The listing builds one solid part. Answer for the finished solid, in the listing's coordinates (mm). Round coordinates to 2 decimals unless told otherwise and drop trailing zeros. Write each loop counter-clockwise with the first axis right and the second up, starting at its lowest first coordinate (ties: lowest second). Pieces come first, ordered by that corner, then holes.
(1) A cutting plane is placed at B-B, the plane y = -50. Give the vertices of the cut face in (x, z), and give its area (3 significant figures).
(2) A cutting plane is placed at C-C, the plane x = 10. Give the vertices of the cut face in (y, z).
(3) This flat-tipped pin is pushed along its axis until it touches: pin 1 Ø3.5 at (x, y) = (10, -70) entering from +Z. Where does it stop, or does it pass through?
(4) A cutting plane is placed at A-A, the plane z = -1.5. Give the vertices of the cut face in (x, y).
(5) A cutting plane is placed at D-D, the plane y = -10. Give the vertices of the cut face in (x, z), and give its area (3 significant figures).
(6) Find the intervals of material crossed by probe 1 along X at (y, z) = (-70, -0.65); probe 2 along Y at (x, z) = (10, -0.7); probe 3 along Y at (x, z) = (8, -1.9), in increasing order.
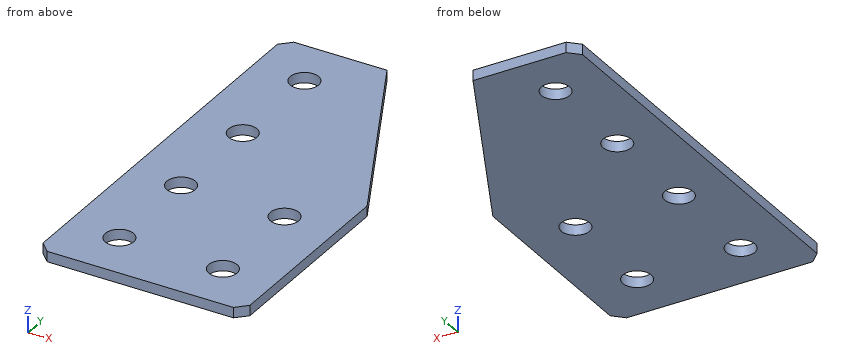
from build123d import *

# Parameters (mm, degrees)
EXTRUDE_1_DEPTH   = 2
HOLE_WIZARD_M51_D = 5.5
CHAMFER_1_SIZE    = 2


with BuildPart() as part:
    # Эскиз1 → Бобышка-Вытянуть1 (new body)
    with BuildSketch(Plane(origin=(0, 0, 0), x_dir=(1, 0, 0), z_dir=(0, 0, -1))):
        Polygon((0, 0), (0, 80), (40, 80), (40, 40), (20, 0), align=None)
    extrude(amount=EXTRUDE_1_DEPTH)

    # Отверстие с зазором M51 (through all)
    with Locations(Plane(origin=(0, 0, -2), x_dir=(1, 0, 0), z_dir=(0, 0, -1))):
        with Locations((10, 70), (10, 50), (10, 30), (10, 10), (30, 70), (30, 50)):
            Hole(HOLE_WIZARD_M51_D / 2)

    # Фаска1
    chamfer_1_edges = [part.edges().sort_by_distance(p)[0] for p in [
        (0, 0, -1),
        (0, -80, -1),
        (40, -80, -1),
    ]]
    chamfer(chamfer_1_edges, length=CHAMFER_1_SIZE)


solid = part.part
Solutions:
1. outline: (0, -2) - (7.25, -2) - (7.25, 0) - (0, 0) - close; (12.75, -2) - (27.25, -2) - (27.25, 0) - (12.75, 0) - close; (32.75, -2) - (40, -2) - (40, 0) - (32.75, 0) - close
1. area: 58.0 mm2
2. outline: (-80, -2) - (-72.75, -2) - (-72.75, 0) - (-80, 0) - close; (-67.25, -2) - (-52.75, -2) - (-52.75, 0) - (-67.25, 0) - close; (-47.25, -2) - (-32.75, -2) - (-32.75, 0) - (-47.25, 0) - close; (-27.25, -2) - (-12.75, -2) - (-12.75, 0) - (-27.25, 0) - close; (-7.25, -2) - (0, -2) - (0, 0) - (-7.25, 0) - close
3. pin 1: passes through
4. outline: (0, -78) - (2, -80) - (38, -80) - (40, -78) - (40, -40) - (20, 0) - (2, 0) - (0, -2) - close; hole circle Ø5.5 at (10, -70); hole circle Ø5.5 at (10, -50); hole circle Ø5.5 at (10, -30); hole circle Ø5.5 at (10, -10); hole circle Ø5.5 at (30, -70); hole circle Ø5.5 at (30, -50)
5. outline: (0, -2) - (7.25, -2) - (7.25, 0) - (0, 0) - close; (12.75, -2) - (25, -2) - (25, 0) - (12.75, 0) - close
5. area: 39.0 mm2
6. probe 1: x = 0 to 7.25, 12.75 to 27.25, 32.75 to 40
6. probe 2: y = -80 to -72.75, -67.25 to -52.75, -47.25 to -32.75, -27.25 to -12.75, -7.25 to 0
6. probe 3: y = -80 to -71.89, -68.11 to -51.89, -48.11 to -31.89, -28.11 to -11.89, -8.11 to 0
